```python
from build123d import *
from OCP.BRepFilletAPI import BRepFilletAPI_MakeChamfer

# Parameters (mm, degrees)
SKETCH1_W           = 101.6
SKETCH1_H           = 50.8
SKETCH1_R           = 0.5
BOSS_EXTRUDE1_DEPTH = 2
SKETCH2_R           = 1.25
SKETCH2_R_2         = 0.5
BOSS_EXTRUDE2_DEPTH = 8
CHAMFER1_SIZE       = 5
CHAMFER1_SIZE2      = 0.437443318


with BuildPart() as part:
    # Sketch1 → Boss-Extrude1 (new body)
    with BuildSketch(Plane(origin=(0, 0, 0), x_dir=(1, 0, 0), z_dir=(0, 1, 0))):
        with Locations((24.438845131, -1.159672083)):
            Rectangle(SKETCH1_W, SKETCH1_H)
        with Locations(Location((-11.121154869, 21.700327917, 0), (0, 0, 270))):
            Circle(SKETCH1_R, mode=Mode.SUBTRACT)
        with Locations(Location((-12.391154869, -24.019672083, 0), (0, 0, 270))):
            Circle(SKETCH1_R, mode=Mode.SUBTRACT)
        with Locations(Location((63.808845131, 21.700327917, 0), (0, 0, 270))):
            Circle(SKETCH1_R, mode=Mode.SUBTRACT)
        with Locations(Location((70.158845131, -24.019672083, 0), (0, 0, 270))):
            Circle(SKETCH1_R, mode=Mode.SUBTRACT)
    extrude(amount=BOSS_EXTRUDE1_DEPTH)

    # Sketch2 → Boss-Extrude2 (add)
    # profile 1 of 4: a face of its own
    with BuildSketch(Plane(origin=(0, 2, 0), x_dir=(1, 0, 0), z_dir=(0, 1, 0))):
        with Locations(Location((-11.121154869, 21.700327917, 0), (0, 0, 270))):
            Circle(SKETCH2_R)
        with Locations(Location((-11.121154869, 21.700327917, 0), (0, 0, 270))):
            Circle(SKETCH2_R_2, mode=Mode.SUBTRACT)
    # profile 2 of 4: a face of its own
    with BuildSketch(Plane(origin=(0, 2, 0), x_dir=(1, 0, 0), z_dir=(0, 1, 0))):
        with Locations(Location((-12.391154869, -24.019672083, 0), (0, 0, 270))):
            Circle(SKETCH2_R)
        with Locations(Location((-12.391154869, -24.019672083, 0), (0, 0, 270))):
            Circle(SKETCH2_R_2, mode=Mode.SUBTRACT)
    # profile 3 of 4: a face of its own
    with BuildSketch(Plane(origin=(0, 2, 0), x_dir=(1, 0, 0), z_dir=(0, 1, 0))):
        with Locations(Location((70.158845131, -24.019672083, 0), (0, 0, 270))):
            Circle(SKETCH2_R)
        with Locations(Location((70.158845131, -24.019672083, 0), (0, 0, 270))):
            Circle(SKETCH2_R_2, mode=Mode.SUBTRACT)
    # profile 4 of 4: a face of its own
    with BuildSketch(Plane(origin=(0, 2, 0), x_dir=(1, 0, 0), z_dir=(0, 1, 0))):
        with Locations(Location((63.808845131, 21.700327917, 0), (0, 0, 270))):
            Circle(SKETCH2_R)
        with Locations(Location((63.808845131, 21.700327917, 0), (0, 0, 270))):
            Circle(SKETCH2_R_2, mode=Mode.SUBTRACT)
    extrude(amount=BOSS_EXTRUDE2_DEPTH)

    # Chamfer1: one chamfer whose edges measure the first distance from different faces: ONE call of the kernel's chamfer builder (chamfer() names one face for all edges)
    chamfer1_edges_1 = [part.edges().sort_by_distance(p)[0] for p in [
        (-11.121154869, 10, -22.950327917),
    ]]
    chamfer1_side_1 = [part.faces().sort_by_distance(p)[0] for p in [
        (-11.121154869, 6, -22.950327917),
    ]]
    chamfer1_edges_2 = [part.edges().sort_by_distance(p)[0] for p in [
        (-12.391154869, 10, 22.769672083),
    ]]
    chamfer1_side_2 = [part.faces().sort_by_distance(p)[0] for p in [
        (-12.391154869, 6, 22.769672083),
    ]]
    chamfer1_edges_3 = [part.edges().sort_by_distance(p)[0] for p in [
        (70.158845131, 10, 22.769672083),
    ]]
    chamfer1_side_3 = [part.faces().sort_by_distance(p)[0] for p in [
        (70.158845131, 6, 22.769672083),
    ]]
    chamfer1_edges_4 = [part.edges().sort_by_distance(p)[0] for p in [
        (63.808845131, 10, -22.950327917),
    ]]
    chamfer1_side_4 = [part.faces().sort_by_distance(p)[0] for p in [
        (63.808845131, 6, -22.950327917),
    ]]
    chamfer1 = BRepFilletAPI_MakeChamfer(part.part.solid().wrapped)
    for e in chamfer1_edges_1:
        chamfer1.Add(CHAMFER1_SIZE, CHAMFER1_SIZE2, e.wrapped, chamfer1_side_1[0].wrapped)  # the first distance lies on this face
    for e in chamfer1_edges_2:
        chamfer1.Add(CHAMFER1_SIZE, CHAMFER1_SIZE2, e.wrapped, chamfer1_side_2[0].wrapped)  # the first distance lies on this face
    for e in chamfer1_edges_3:
        chamfer1.Add(CHAMFER1_SIZE, CHAMFER1_SIZE2, e.wrapped, chamfer1_side_3[0].wrapped)  # the first distance lies on this face
    for e in chamfer1_edges_4:
        chamfer1.Add(CHAMFER1_SIZE, CHAMFER1_SIZE2, e.wrapped, chamfer1_side_4[0].wrapped)  # the first distance lies on this face
    add(Compound.cast(chamfer1.Shape()), mode=Mode.REPLACE)


solid = part.part
```
Geometry: final body of the model. Coordinates: model frame, mm. A direction names the side the tool comes from. Coordinates: 2 decimals unless noted, no trailing zeros. Loops run counter-clockwise (first coordinate to the right, second up) from the corner with the lowest first, then second, coordinate; pieces in that order, holes last. Notation, with made-up numbers: (-2.75, 49) -> (21.25, 49) arc R6 cw to (21.25, 60) -> close; hole circle Ø1 at (19.25, -38). An arc over 180 degrees is marked (long way). Use a Markdown table: item, result. Add a question column.
(1) Section query A-A, the plane y = 7.25. Return loops of the section in (x, z).
(2) Section query C-C, the plane z = -11.5. Return loops of the section in (x, y).
(3) Mould query, pull axis X, two halves, no side actions, for faces 1 (the cylindrical face through (62.59, 3.48, -21.97)), 2 (the flat face through (-26.361, 1, 2)), 3 (the flat face through (24, 1, 26.56)). Classes: pulls with the +X half, pulls with the -X half, needs draft (parallel to the pull), parting line crosses it, or undercut.
(4) Section query B-B, the plane x = 43.5. Return loops of the section in (y, z), plus the area to 3 significant figures.
(5) Line query: line 1 along X through (y, z) = (4.5, 24); line 2 along Y through (x, z) = (23.5, -18); line 3 along Z through (x, y) = (-12.5, 5.5). Output: solid intervals per line, ascending.
(6) Pin query (flat end, axial travel): pin 1 Ø1 at (x, z) = (11, -13) entering from +Y. Return the tip coordinate at first contact, or that it passes through.
(7) Access query for faces 4 (the cylindrical face through (-11.07, 3.48, -22.95)), 5 (the flat face through (24, 1, -24.24)). Directions: +Z, -Z, +X, -X, +Y, -Y. A direction counts if a zero-diameter tool reaches every point of the face in a straight line with its end or side. Return the directions, or none.
Answer:
| question | item | result |
|---|---|---|
| 1 | outline | circle Ø2.11 at (-12.39, 24.02); circle Ø2.11 at (-11.12, -21.7); circle Ø2.11 at (63.81, -21.7); circle Ø2.11 at (70.16, 24.02); hole circle Ø1 at (-12.39, 24.02); hole circle Ø1 at (-11.12, -21.7); hole circle Ø1 at (63.81, -21.7); hole circle Ø1 at (70.16, 24.02) |
| 2 | outline | (-26.36, 0) -> (75.24, 0) -> (75.24, 2) -> (-26.36, 2) -> close |
| 3 | face 1 | undercut |
| 3 | face 2 | pulls with the -X half |
| 3 | face 3 | needs draft |
| 4 | outline | (0, -24.24) -> (2, -24.24) -> (2, 26.56) -> (0, 26.56) -> close |
| 4 | area | 102 mm^2 |
| 5 | line 1 | x = -13.64 to -12.89, -11.89 to -11.14, 68.91 to 69.66, 70.66 to 71.41 |
| 5 | line 2 | y = 0 to 2 |
| 5 | line 3 | z = 22.82 to 23.53, 24.51 to 25.22 |
| 6 | pin 1 | stops at y = 2 |
| 7 | face 4 | +Y |
| 7 | face 5 | -Z, +X, -X, +Y, -Y |
